The model under review builds one solid part; all positions refer to its coordinate system, in mm. Face numbers are marked on the shaded views. A direction names the side the tool comes from. Give positions to 0.01 mm unless a question says otherwise; leave off trailing zeros. Write each loop counter-clockwise with the first axis right and the second up, starting at its lowest first coordinate (ties: lowest second). Pieces come first, ordered by that corner, then holes.
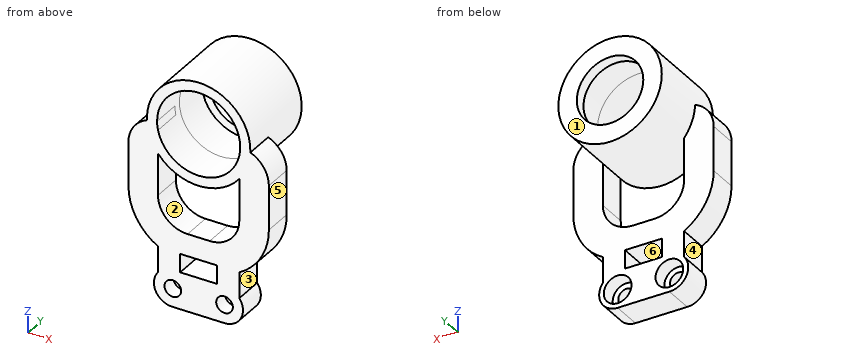
from build123d import *

# Parameters (mm, degrees)
SKETCH005_R             = 14
SKETCH005_R_2           = 11.25
PAD005_DEPTH            = 20
SKETCH006_R             = 14
SKETCH006_R_2           = 9
PAD006_DEPTH            = 3
SKETCH007_W             = 10
SKETCH007_H             = 5
PAD007_DEPTH            = 8
HOLE_D                  = 4.5
HOLE_DEPTH              = 25
HOLE_CBORE_D            = 7.5
HOLE_CBORE_DEPTH        = 4
SKETCH032_R             = 11.25
POCKET002_DEPTH         = 10
BODY002_PLACEMENT_ANGLE = 180


with BuildPart() as part:
    # Sketch005 → Pad005 (new body)
    with BuildSketch(Plane.XZ):
        Circle(SKETCH005_R)
        Circle(SKETCH005_R_2, mode=Mode.SUBTRACT)
    extrude(amount=PAD005_DEPTH)

    # Sketch006 (on Face3 of Pad005) → Pad006 (join)
    with BuildSketch(Plane(origin=(0, 0, 0), x_dir=(1, 0, 0), z_dir=(0, 1, 0))):
        Circle(SKETCH006_R)
        Circle(SKETCH006_R_2, mode=Mode.SUBTRACT)
    extrude(amount=PAD006_DEPTH)

    # Sketch007 (on Face3 of Pad006) → Pad007 (join)
    with BuildSketch(Plane.XZ.offset(20)):
        with BuildLine():
            Line((-11, 20), (-11, 0))
            ThreePointArc((-19, 8), (-16.656854, 2.343146), (-11, 0))
            Line((-19, 8), (-19, 20))
            ThreePointArc((-11, 34), (-16.892531, 28.081446), (-19, 20))
            Line((-11, 34), (-11, 41))
            ThreePointArc((-7, 49), (-11.472136, 46.236068), (-11, 41))
            Line((-7, 49), (7, 49))
            ThreePointArc((11, 40.856406), (11.600717, 46.205633), (7, 49))
            Line((11, 33.856406), (11, 40.856406))
            ThreePointArc((19, 20), (16.856406, 28), (11, 33.856406))
            Line((19, 20), (19, 8))
            ThreePointArc((11, 0), (16.656854, 2.343146), (19, 8))
            Line((11, 0), (11, 20))
            ThreePointArc((11, 20), (8.656855, 25.656854), (3.000001, 28))
            Line((-2.999999, 28), (3.000001, 28))
            ThreePointArc((-2.999999, 28), (-8.656854, 25.656855), (-11, 20))
        make_face()
        with Locations((0, 36.5)):
            Rectangle(SKETCH007_W, SKETCH007_H, mode=Mode.SUBTRACT)
    extrude(amount=-PAD007_DEPTH)

    # Hole
    with Locations(Plane(origin=(0, -12, 0), x_dir=(1, 0, 0), z_dir=(0, 1, 0))):
        with Locations((-7, -44), (7, -44)):
            CounterBoreHole(HOLE_D / 2, HOLE_CBORE_D / 2, HOLE_CBORE_DEPTH, depth=HOLE_DEPTH)

    # Sketch032 (on Face7 of Hole) → Pocket002 (cut)
    with BuildSketch(Plane.XZ.offset(20)):
        Circle(SKETCH032_R)
    extrude(amount=-POCKET002_DEPTH, mode=Mode.SUBTRACT)


with BuildPart() as part_1:
    # Body002 placement: moved
    add(part.part.moved(Location((19, 198, 62))).rotate(Axis((19, 198, 62), (0, 1, 0)), BODY002_PLACEMENT_ANGLE))


solid = part_1.part
1) The part is to be moulded in two halves that separate along X. For the marked faces 1, 2, 3 and 4, say which applies: +X half, -X half, draft (parallel to the pull), parting line (faces both ways), or undercut.
2) To check wall thickness, follow probe 1 along X at (y, z) = (185.25, 47.5); probe 2 along X at (y, z) = (184, 52.5); probe 3 along Z at (x, y) = (15, 180.5). State the ranges of each line that lie inside material, in increasing order.
3) Consider section D-D, the plane y = 191.5. Give the boundary of the cut face in (x, z), then the cut area to 3 significant figures.
4) Consider section B-B, the plane z = 18. Give the boundary of the cut face in (x, y), then the cut area to 3 significant figures.
5) Insertion check: pin 1 (8.5 mm diameter, centred on x = 26, z = 18, fed in from +Y); pin 2 (2 mm diameter, centred on x = 5.5, y = 197, fed in from -Z); pin 3 (3 mm diameter, centred on x = 25.5, y = 197.5, fed in from -Z). Each pin has a flat end and moves straight along its axis. Give the tip position at first contact, or say it passes through.
6) Consider section C-C, the plane z = 68. Give the boundary of the cut face in (x, y), then the cut area to 3 significant figures.
7) Tool access review of the marked faces 5 and 6: name each direction out of +Z, -Z, +X, -X, +Y, -Y from which nothing blocks a thin tool from reaching the whole face with its end or side.
8) Consider section A-A, the plane x = 19. Give the boundary of the cut face in (y, z).
Answer block:
1. face 1: draft
1. face 2: undercut
1. face 3: +X half
1. face 4: -X half
2. probe 1: x = 0 to 8, 30 to 38
2. probe 2: x = 0 to 8, 8.72 to 12.97, 25.03 to 29.28, 30 to 38
2. probe 3: z = 13 to 23, 28 to 34.06, 48.58 to 51.49, 72.51 to 75.42
3. outline: circle Ø28 at (19, 62); hole circle Ø22.5 at (19, 62)
3. area: 218 mm2
4. outline: (6.89, 178) - (9.75, 178) - (9.75, 182) - (8.25, 182) - (8.25, 186) - (6.89, 186) - close; (14.25, 178) - (23.75, 178) - (23.75, 182) - (22.25, 182) - (22.25, 186) - (15.75, 186) - (15.75, 182) - (14.25, 182) - close; (28.25, 178) - (31, 178) - (31, 186) - (29.75, 186) - (29.75, 182) - (28.25, 182) - close
4. area: 96.9 mm2
5. pin 1: stops at y = 186
5. pin 2: stops at z = 55.7
5. pin 3: stops at z = 48.92
6. outline: (6.35, 178) - (9.48, 178) - (9.48, 198) - (12.29, 198) - (12.29, 201) - (6.35, 201) - close; (25.71, 198) - (28.52, 198) - (28.52, 178) - (31.65, 178) - (31.65, 201) - (25.71, 201) - close
6. area: 161 mm2
7. face 5: +Z, -Z, +X, +Y, -Y
7. face 6: +Y, -Y
8. outline: (178, 13) - (186, 13) - (186, 23) - (178, 23) - close; (178, 28) - (186, 28) - (186, 34) - (178, 34) - close; (178, 48) - (201, 48) - (201, 53) - (198, 53) - (198, 50.75) - (178, 50.75) - close; (178, 73.25) - (198, 73.25) - (198, 71) - (201, 71) - (201, 76) - (178, 76) - close
